```python
from build123d import *

# Parameters (mm, degrees)
SKETCH1_R                = 9.25
SKETCH1_R_2              = 7.95
BOSS_EXTRUDE1_DEPTH      = 5
BOSS_EXTRUDE2_START      = 5
SKETCH3_R                = 8.25
SKETCH3_R_2              = 6.95
BOSS_EXTRUDE2_DEPTH      = 2.5
BOSS_EXTRUDE2_DEPTH_BACK = 1
SKETCH4_R                = 8.25
BOSS_EXTRUDE3_DEPTH      = 1.3
SKETCH5_R                = 4.03
SKETCH5_R_2              = 2.38
BOSS_EXTRUDE4_DEPTH      = 6.7
SKETCH5_2_R              = 2.38
CUT_EXTRUDE1_DEPTH       = 15.697448758
SKETCH6_W                = 4.65
SKETCH6_H                = 2
CUT_EXTRUDE2_DEPTH       = 16.333786225
CIRPATTERN1_COUNT        = 3
SKETCH7_R                = 2.38
BOSS_EXTRUDE5_DEPTH      = 0.4
BOSS_EXTRUDE6_DEPTH      = 2.8
CIRPATTERN2_COUNT        = 3


with BuildPart() as part:
    # Sketch1 → Boss-Extrude1 (new body)
    with BuildSketch(Plane.XY):
        Circle(SKETCH1_R)
        Circle(SKETCH1_R_2, mode=Mode.SUBTRACT)
    extrude(amount=BOSS_EXTRUDE1_DEPTH)

    # Sketch3 → Boss-Extrude2 (add, two sides)
    with BuildSketch(Plane.XY.offset(BOSS_EXTRUDE2_START)) as boss_extrude2_sk:
        Circle(SKETCH3_R)
        Circle(SKETCH3_R_2, mode=Mode.SUBTRACT)
    extrude(amount=BOSS_EXTRUDE2_DEPTH)
    extrude(boss_extrude2_sk.sketch, amount=-BOSS_EXTRUDE2_DEPTH_BACK)

    # Sketch4 → Boss-Extrude3 (add)
    with BuildSketch(Plane.XY.offset(7.5)):
        Circle(SKETCH4_R)
    extrude(amount=-BOSS_EXTRUDE3_DEPTH)

    # Sketch5 → Boss-Extrude4 (add)
    with BuildSketch(Plane(origin=(0, 0, 6.2), x_dir=(-1, 0, 0), z_dir=(0, 0, -1))):
        with Locations(Location((0, 0, 0), (0, 0, 180))):
            Circle(SKETCH5_R)
        with Locations(Location((0, 0, 0), (0, 0, 180))):
            Circle(SKETCH5_R_2, mode=Mode.SUBTRACT)
    extrude(amount=BOSS_EXTRUDE4_DEPTH)

    # Sketch5<2> → Cut-Extrude1 (cut, through all)
    with BuildSketch(Plane(origin=(0, 0, 6.2), x_dir=(-1, 0, 0), z_dir=(0, 0, -1))):
        with Locations(Location((0, 0, 0), (0, 0, 180))):
            Circle(SKETCH5_2_R)
    extrude(amount=-CUT_EXTRUDE1_DEPTH, mode=Mode.SUBTRACT)

    # Sketch6 → Cut-Extrude2 (cut, through all)
    with BuildSketch(Plane.XY.offset(7.5)):
        with Locations((0, 4.83)):
            Rectangle(SKETCH6_W, SKETCH6_H)
    cut_extrude2 = extrude(amount=-CUT_EXTRUDE2_DEPTH, mode=Mode.SUBTRACT)

    # CirPattern1: Cut-Extrude2 ×3 about axis
    cirpattern1_axis = Axis((0, 0, 0), (0, 0, 1))
    for i in range(1, CIRPATTERN1_COUNT):
        add(cut_extrude2.rotate(cirpattern1_axis, i * 360 / CIRPATTERN1_COUNT), mode=Mode.SUBTRACT)

    # Sketch7 → Boss-Extrude5 (add)
    with BuildSketch(Plane.XY.offset(7.5)):
        Polygon((-1.922576396, -3.33), (1.922576396, -3.33), (3.845152793, 0), (1.922576396, 3.33), (-1.922576396, 3.33), (-3.845152793, 0), align=None)
        Circle(SKETCH7_R, mode=Mode.SUBTRACT)
    extrude(amount=BOSS_EXTRUDE5_DEPTH)

    # Sketch8 → Boss-Extrude6 (add)
    with BuildSketch(Plane.XY.offset(7.5)):
        with BuildLine():
            Line((3.636428104, -5.361521766), (1.904377296, -4.361521766))
            ThreePointArc((1.904377296, -4.361521766), (0, -4.75915171), (-1.904377296, -4.361521766))
            Line((-1.904377296, -4.361521766), (-3.636428104, -5.361521766))
            Line((-3.636428104, -5.361521766), (-2.130298289, -7.970215129))
            ThreePointArc((-2.130298289, -7.970215129), (1.516159822, -8.109485766), (4.865989618, -6.662180201))
            Line((4.865989618, -6.662180201), (3.636428104, -5.361521766))
        make_face()
    boss_extrude6 = extrude(amount=BOSS_EXTRUDE6_DEPTH)

    # CirPattern2: Boss-Extrude6 ×3 about axis
    cirpattern2_axis = Axis((0, 0, 0), (0, 0, 1))
    for i in range(1, CIRPATTERN2_COUNT):
        add(boss_extrude6.rotate(cirpattern2_axis, i * 360 / CIRPATTERN2_COUNT))


solid = part.part
```
Geometry check sheet. Reference: the model listing, model coordinates, mm. A direction names the side the tool comes from. Round coordinates to 2 decimals unless told otherwise and drop trailing zeros. Order: outer loops, then holes, each group sorted by start corner. A loop starts at its lowest first (then second) coordinate and runs counter-clockwise, first axis right, second up. Notation, with made-up numbers: (52, -21) -> (77, -21) arc R31 cw to (77, 4) -> close; hole circle Ø3 at (84, -20.75). An arc over 180 degrees is marked (long way). Return JSON: item names as keys, results as strings. Group by question number.
Q1. Section check A-A, the plane z = 1. Record the boundary of the cut face in (x, y), plus the area to 3 significant figures.
Q2. Material ranges on probe 1 along Y at (x, z) = (0, 4.25); probe 2 along Y at (x, z) = (0, 1.2); probe 3 along X at (y, z) = (0, 5.5), recorded low to high. Write a range as from..to.
Q3. Tool access check on faces 5 (the cylindrical face through (-4.135, 2.356, 8.88)), 6 (the flat face through (0, 5.83, 7)), 7 (the cylindrical face through (3.47, 2.05, 2.9)). Record the directions out of +Z, -Z, +X, -X, +Y, -Y that give a thin tool (end or side, any length) a straight path to the whole face; none if there is none.
Q4. Release check for a two-part mould opening along X. For faces 1 (the cylindrical face through (4.11, 2.4, 8.88)), 2 (the flat face through (-5, -3, 7)), 3 (the flat face through (-4, 5.83, 9)), 4 (the flat face through (4.26, -6.02, 8.88)) record: released by +X, released by -X, zero draft, split by the parting line, or undercut.
Q5. Gauge pin test, flat ends, axial feed: pin 1 (2 mm diameter, centred on y = -5, z = 1.5, fed in from +X); pin 2 (1 mm diameter, centred on y = 5.5, z = 8.5, fed in from +X); pin 3 (1.4 mm diameter, centred on x = 1, z = 6.5, fed in from -Y). Record the tip position at first contact, or that the pin passes through.
Q6. Section check B-B, the plane x = 0. Count the separate pieces of the cut face and the enclosed holes in it, plus the area to 3 significant figures.
Q7. Section check D-D, the plane x = -5.25. Record the boundary of the cut face in (y, z).
Numbers:
{
 "1": {"outline": "circle Ø18.5 at (0, 0); (-3.94, -0.83) -> (-2.69, -3) arc R4.03 ccw to (2.69, -3) -> (3.94, -0.83) arc R4.03 ccw to (1.25, 3.83) -> (-1.25, 3.83) arc R4.03 ccw to start; hole circle Ø15.9 at (0, 0); hole circle Ø4.76 at (0, 0)", "area": "102 mm^2"},
 "2": {"probe 1": "-9.25..-6.95, -4.03..-2.38, 2.38..3.83, 6.95..9.25", "probe 2": "-9.25..-7.95, -4.03..-2.38, 2.38..3.83, 7.95..9.25", "probe 3": "-8.25..-6.95, -4.03..-2.38, 2.38..4.03, 6.95..8.25"},
 "3": {"face 5": "+Z", "face 6": "+Z, -Z", "face 7": "-Z"},
 "4": {"face 1": "undercut", "face 2": "undercut", "face 3": "zero draft", "face 4": "released by +X"},
 "5": {"pin 1": "x = 8.34", "pin 2": "x = 6.56", "pin 3": "y = -8.24"},
 "6": {"separate pieces": "3", "enclosed holes": "0", "area": "62.1 mm^2"},
 "7": {"outline": "(-7.62, 0) -> (-5.97, 0) -> (-5.97, 4) -> (-4.55, 4) -> (-4.55, 6.2) -> (-2.57, 6.2) -> (-2.57, 7.5) -> (-6.36, 7.5) -> (-6.36, 5) -> (-7.62, 5) -> close; (-0.35, 6.2) -> (4.55, 6.2) -> (4.55, 4) -> (5.97, 4) -> (5.97, 0) -> (7.62, 0) -> (7.62, 5) -> (6.36, 5) -> (6.36, 7.5) -> (5.83, 7.5) -> (5.83, 10.3) -> (0.23, 10.3) -> (0.23, 7.5) -> (-0.35, 7.5) -> close"}
}
